The listing builds one solid part. Answer for the finished solid, in the listing's coordinates (mm). Coordinates: 2 decimals unless noted, no trailing zeros. Write each loop counter-clockwise with the first axis right and the second up, starting at its lowest first coordinate (ties: lowest second). Pieces come first, ordered by that corner, then holes. Notation, with made-up numbers: M -3,75.25 L 7,75.25 A20 ccw 7,82.25 Z; hole C 0,-4 d5. An arc over 180 degrees is marked long. Answer as a JSON object with one key per item and string values. Group by question number.
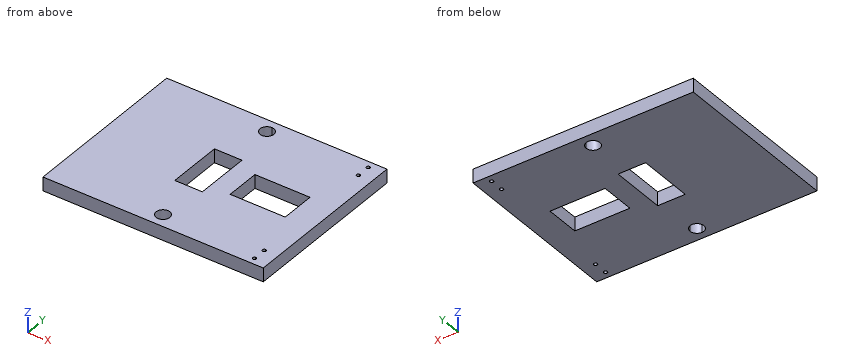
from build123d import *

# Parameters (mm, degrees)
F0_W     = 12.7
F0_H     = 15.875
F1_DEPTH = 6.35
F2_R     = 0.8255
F2_W     = 6.35
F2_H     = 12.7
F3_DEPTH = 25.4


with BuildPart() as f1:
    # F0 (on Top) → F1 (new body)
    with BuildSketch(Plane.XY):
        with BuildLine():
            Line((0, -12.7), (0, 0))
            Line((0, 0), (-6.35, 0))
            Line((-6.35, 0), (-6.35, -2.3495))
            ThreePointArc((-6.35, -2.3495), (-5.766283, -2.591283), (-5.5245, -3.175))
            ThreePointArc((-5.5245, -3.175), (-5.766283, -3.758717), (-6.35, -4.0005))
            Line((-6.35, -4.0005), (-6.35, -8.6995))
            ThreePointArc((-6.35, -8.6995), (-5.766283, -8.941283), (-5.5245, -9.525))
            ThreePointArc((-5.5245, -9.525), (-5.766283, -10.108717), (-6.35, -10.3505))
            Line((-6.35, -10.3505), (-6.35, -12.7))
            Line((-6.35, -12.7), (0, -12.7))
        make_face()
        with BuildLine():
            Line((-6.35, -2.3495), (-6.35, 0))
            Line((-6.35, 0), (-12.7, 0))
            Line((-12.7, 0), (-12.7, -12.7))
            Line((-12.7, -12.7), (-6.35, -12.7))
            Line((-6.35, -12.7), (-6.35, -10.3505))
            ThreePointArc((-6.35, -10.3505), (-7.1755, -9.525), (-6.35, -8.6995))
            Line((-6.35, -8.6995), (-6.35, -4.0005))
            ThreePointArc((-6.35, -4.0005), (-7.1755, -3.175), (-6.35, -2.3495))
        make_face()
        with BuildLine():
            ThreePointArc((-47.625, -6.35), (-48.554936, -4.104936), (-50.8, -3.175))
            ThreePointArc((-50.8, -3.175), (-53.045064, -8.595064), (-47.625, -6.35))
        make_face()
        with BuildLine():
            ThreePointArc((-47.625, -73.025), (-53.045064, -70.779936), (-50.8, -76.2))
            ThreePointArc((-50.8, -76.2), (-48.554936, -75.270064), (-47.625, -73.025))
        make_face()
        Polygon((0, -31.75), (0, -12.7), (-6.35, -12.7), (-12.7, -12.7), (-12.7, 0), (-50.8, 0), (-101.6, 0), (-101.6, -79.375), (-50.8, -79.375), (-12.7, -79.375), (-12.7, -66.675), (-6.35, -66.675), (0, -66.675), (0, -47.625), (-12.7, -47.625), (-38.1, -47.625), (-38.1, -31.75), (-12.7, -31.75), align=None)
        with BuildLine():
            ThreePointArc((-47.625, -73.025), (-48.554936, -75.270064), (-50.8, -76.2))
            ThreePointArc((-50.8, -76.2), (-53.045064, -70.779936), (-47.625, -73.025))
        make_face(mode=Mode.SUBTRACT)
        with BuildLine():
            ThreePointArc((-47.625, -6.35), (-53.045064, -8.595064), (-50.8, -3.175))
            ThreePointArc((-50.8, -3.175), (-48.554936, -4.104936), (-47.625, -6.35))
        make_face(mode=Mode.SUBTRACT)
        with Locations((-6.35, -39.6875)):
            Rectangle(F0_W, F0_H)
        with BuildLine():
            Line((0, -79.375), (0, -66.675))
            Line((0, -66.675), (-6.35, -66.675))
            Line((-6.35, -66.675), (-6.35, -69.0245))
            ThreePointArc((-6.35, -69.0245), (-5.766283, -69.266283), (-5.5245, -69.85))
            ThreePointArc((-5.5245, -69.85), (-5.766283, -70.433717), (-6.35, -70.6755))
            Line((-6.35, -70.6755), (-6.35, -75.3745))
            ThreePointArc((-6.35, -75.3745), (-5.766283, -75.616283), (-5.5245, -76.2))
            ThreePointArc((-5.5245, -76.2), (-5.766283, -76.783717), (-6.35, -77.0255))
            Line((-6.35, -77.0255), (-6.35, -79.375))
            Line((-6.35, -79.375), (0, -79.375))
        make_face()
        with BuildLine():
            Line((-6.35, -69.0245), (-6.35, -66.675))
            Line((-6.35, -66.675), (-12.7, -66.675))
            Line((-12.7, -66.675), (-12.7, -79.375))
            Line((-12.7, -79.375), (-6.35, -79.375))
            Line((-6.35, -79.375), (-6.35, -77.0255))
            ThreePointArc((-6.35, -77.0255), (-7.1755, -76.2), (-6.35, -75.3745))
            Line((-6.35, -75.3745), (-6.35, -70.6755))
            ThreePointArc((-6.35, -70.6755), (-7.1755, -69.85), (-6.35, -69.0245))
        make_face()
    extrude(amount=F1_DEPTH)

    # F2 (on face) → F3 (cut)
    with BuildSketch(Plane.XY.offset(6.35)):
        with Locations((-6.35, -3.175)):
            Circle(F2_R)
        with Locations((-6.35, -9.525)):
            Circle(F2_R)
        with Locations((-50.673, -33.3375)):
            Rectangle(F2_W, F2_H)
        Polygon((-53.848, -39.6875), (-53.848, -26.9875), (-60.198, -26.9875), (-60.198, -52.3875), (-47.498, -52.3875), (-47.498, -39.6875), align=None)
    extrude(amount=-F3_DEPTH, mode=Mode.SUBTRACT)


solid = f1.part
Item 1: A cutting plane is placed at C-C, the plane y = -43. Write down the section's boundary in (x, z), and give its area (3 significant figures).
Item 2: Consider L1, parallel to X at y = -45.5, z = 3; L2, parallel to X at y = -6, z = 2.25; L3, parallel to Y at x = -37.5, z = 5.5 (3 decimals). Determine where each line is inside the solid, lowest interval first. Write a range as from..to.
Item 3: A cutting plane is placed at A-A, the plane z = 1.5. State how many separate pieces and enclosed holes the cut face has, and give its area (3 significant figures).
Item 4: A cutting plane is placed at B-B, the plane x = -37. Write down the section's boundary in (y, z) (3 decimals), and give its area (3 significant figures).
Answer:
{
 "1": {"outline": "M -101.6,0 L -60.2,0 L -60.2,6.35 L -101.6,6.35 Z; M -47.5,0 L -38.1,0 L -38.1,6.35 L -47.5,6.35 Z; M -12.7,0 L 0,0 L 0,6.35 L -12.7,6.35 Z", "area": "403 mm2"},
 "2": {"L1": "-101.6..-60.2, -47.5..-38.1, -12.7..0", "L2": "-101.6..-53.96, -47.64..0", "L3": "-79.375..-47.625, -31.75..0"},
 "3": {"separate pieces": "1", "enclosed holes": "8", "area": "7,270 mm2"},
 "4": {"outline": "M -79.375,0 L -47.625,0 L -47.625,6.35 L -79.375,6.35 Z; M -31.75,0 L 0,0 L 0,6.35 L -31.75,6.35 Z", "area": "403 mm2"}
}
